from build123d import *

# Parameters (mm, degrees)
SKETCH1_W               = 63.5
SKETCH1_H               = 63.5
BOSS_EXTRUDE1_DEPTH     = 5
SKETCH2_W               = 36.5
SKETCH2_H               = 36.5
SKETCH2_W_2             = 26.5
SKETCH2_H_2             = 26.5
BOSS_EXTRUDE2_DEPTH     = 60
SKETCH13_W              = 13.5
SKETCH13_H              = 4
BOSS_EXTRUDE3_DEPTH     = 60
CUT_EXTRUDE1_DEPTH      = 81.059680864
CUT_EXTRUDE1_DEPTH_BACK = 81.059680864
SKETCH15_W              = 13.5
SKETCH15_H              = 4
BOSS_EXTRUDE4_DEPTH     = 60
CUT_EXTRUDE3_DEPTH      = 81.059680864
CUT_EXTRUDE3_DEPTH_BACK = 81.059680864
SKETCH17_W              = 4
SKETCH17_H              = 13.5
BOSS_EXTRUDE5_DEPTH     = 60
CUT_EXTRUDE4_DEPTH      = 81.188668152
CUT_EXTRUDE4_DEPTH_BACK = 81.188668152
SKETCH21_R              = 3.175
CUT_EXTRUDE7_DEPTH      = 20


with BuildPart() as part:
    # Sketch1 → Boss-Extrude1 (new body)
    with BuildSketch(Plane(origin=(0, 0, 0), x_dir=(1, 0, 0), z_dir=(0, 1, 0))):
        Rectangle(SKETCH1_W, SKETCH1_H)
    extrude(amount=BOSS_EXTRUDE1_DEPTH)

    # Sketch2 → Boss-Extrude2 (add)
    with BuildSketch(Plane(origin=(0, 5, 0), x_dir=(1, 0, 0), z_dir=(0, 1, 0))):
        Rectangle(SKETCH2_W, SKETCH2_H)
        Rectangle(SKETCH2_W_2, SKETCH2_H_2, mode=Mode.SUBTRACT)
    extrude(amount=BOSS_EXTRUDE2_DEPTH)

    # Sketch13 → Boss-Extrude3 (add)
    with BuildSketch(Plane(origin=(0, 5, 0), x_dir=(1, 0, 0), z_dir=(0, 1, 0))):
        with Locations((-25, -0.55)):
            Rectangle(SKETCH13_W, SKETCH13_H)
    extrude(amount=BOSS_EXTRUDE3_DEPTH)

    # Sketch14 → Cut-Extrude1 (cut, two sides: drawn at the far end of the back side and taken through both)
    with BuildSketch(Plane.XY.offset(2.55).offset(-CUT_EXTRUDE1_DEPTH_BACK)):
        Polygon((-72.29949978, -175.219999022), (-31.75, 5), (-18.25, 65), (22.29949978, 245.219999022), (-338.140498264, 326.318998582), (-432.739497824, -94.120999462), align=None)
    extrude(amount=CUT_EXTRUDE1_DEPTH + CUT_EXTRUDE1_DEPTH_BACK, mode=Mode.SUBTRACT)

    # Sketch15 → Boss-Extrude4 (add)
    with BuildSketch(Plane(origin=(0, 5, 0), x_dir=(1, 0, 0), z_dir=(0, 1, 0))):
        with Locations((25, -0.55)):
            Rectangle(SKETCH15_W, SKETCH15_H)
    extrude(amount=BOSS_EXTRUDE4_DEPTH)

    # Sketch16 → Cut-Extrude3 (cut, two sides: drawn at the far end of the back side and taken through both)
    with BuildSketch(Plane.XY.offset(2.55).offset(-CUT_EXTRUDE3_DEPTH_BACK)):
        Polygon((72.29949978, -175.219999022), (31.75, 5), (18.25, 65), (-22.29949978, 245.219999022), (338.140498264, 326.318998582), (432.739497824, -94.120999462), align=None)
    extrude(amount=CUT_EXTRUDE3_DEPTH + CUT_EXTRUDE3_DEPTH_BACK, mode=Mode.SUBTRACT)

    # Sketch17 → Boss-Extrude5 (add)
    with BuildSketch(Plane(origin=(0, 5, 0), x_dir=(1, 0, 0), z_dir=(0, 1, 0))):
        with Locations((-0.85, -25)):
            Rectangle(SKETCH17_W, SKETCH17_H)
    extrude(amount=BOSS_EXTRUDE5_DEPTH)

    # Sketch18 → Cut-Extrude4 (cut, two sides: drawn at the far end of the back side and taken through both)
    with BuildSketch(Plane.ZY.offset(2.85).offset(-CUT_EXTRUDE4_DEPTH_BACK)):
        Polygon((72.29949978, -175.219999022), (31.75, 5), (18.25, 65), (-22.29949978, 245.219999022), (338.140498264, 326.318998582), (432.739497824, -94.120999462), align=None)
    extrude(amount=CUT_EXTRUDE4_DEPTH + CUT_EXTRUDE4_DEPTH_BACK, mode=Mode.SUBTRACT)

    # Sketch21 → Cut-Extrude7 (cut)
    with BuildSketch(Plane(origin=(0, 0, -18.25), x_dir=(-1, 0, 0), z_dir=(0, 0, -1))):
        with Locations((0, 17.739365868)):
            Circle(SKETCH21_R)
        with Locations((0, 47.466444019)):
            Circle(SKETCH21_R)
    extrude(amount=-CUT_EXTRUDE7_DEPTH, mode=Mode.SUBTRACT)


solid = part.part
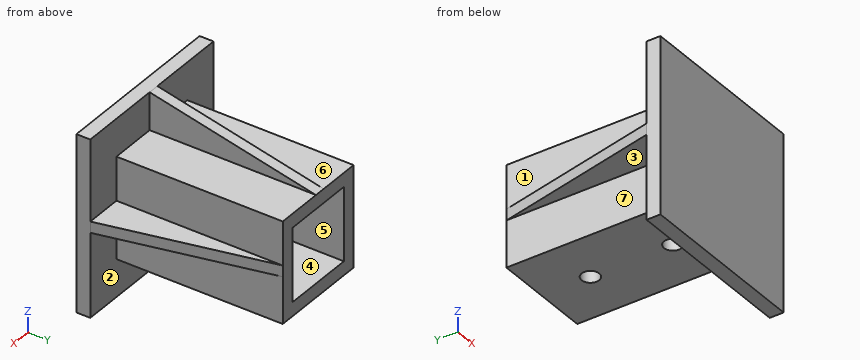
Source: CAD feature listing. Evaluate the final solid. Frame: model axes, mm. Face numbers are marked on the shaded views. A direction names the side the tool comes from. Give positions to 0.01 mm unless a question says otherwise; leave off trailing zeros. Write each loop counter-clockwise with the first axis right and the second up, starting at its lowest first coordinate (ties: lowest second). Pieces come first, ordered by that corner, then holes. Notation, with made-up numbers: M 73.25,4.25 L 120.25,4.25 A14 cw 120.25,26.25 Z; hole C 42,70 d10. An arc over 180 degrees is marked long. Answer as a JSON object with one key per item and string values.
Q1. Ray query, line 1 along Y through (x, z) = (0, -14); line 2 along X through (y, z) = (34, 12). Return the intervals inside material, ascending.
Geometry check:
{"line 1": "y = 0 to 14.56, 20.91 to 44.29, 50.64 to 65", "line 2": "x = -18.25 to -13.25, 13.25 to 18.25"}
Q2. Cut plane C-C, the plane z = -12. Return the cut outline in (x, y).
Geometry check:
{"outline": "M -31.75,0 L 31.75,0 L 31.75,5 L 18.25,5 L 18.25,65 L 13.25,65 L 13.25,5 L -13.25,5 L -13.25,65 L -18.25,65 L -18.25,5 L -31.75,5 Z"}
Q3. Access query for the marked faces 1, 2, 3 and 4. Directions: +Z, -Z, +X, -X, +Y, -Y. A direction counts if a zero-diameter tool reaches every point of the face in a straight line with its end or side. Return the directions, or none.
Geometry check:
{"face 1": "+Z, -X, +Y", "face 2": "-Z, +Y", "face 3": "-Z, -X, +Y", "face 4": "+Y"}
Q4. Cut plane B-B, the plane x = -16.5. Return the cut outline in (y, z), then the cut area to 3 significant figures.
Geometry check:
{"outline": "M 0,-31.75 L 5,-31.75 L 5,-18.25 L 65,-18.25 L 65,18.25 L 5,18.25 L 5,31.75 L 0,31.75 Z", "area": "2,510 mm^2"}
Q5. Cut plane A-A, the plane y = 41. Return the cut outline in (x, z).
Geometry check:
{"outline": "M -23.65,-1.45 L -18.25,-1.45 L -18.25,-18.25 L 18.25,-18.25 L 18.25,-1.45 L 23.65,-1.45 L 23.65,2.55 L 18.25,2.55 L 18.25,18.25 L 1.15,18.25 L 1.15,23.65 L -2.85,23.65 L -2.85,18.25 L -18.25,18.25 L -18.25,2.55 L -23.65,2.55 Z; hole M -13.25,-13.25 L 13.25,-13.25 L 13.25,13.25 L -13.25,13.25 Z"}
Q6. Cut plane D-D, the plane x = 0. Return the cut outline in (y, z).
Geometry check:
{"outline": "M 0,-31.75 L 5,-31.75 L 5,-18.25 L 14.56,-18.25 L 14.56,-13.25 L 5,-13.25 L 5,13.25 L 65,13.25 L 65,18.25 L 5,31.75 L 0,31.75 Z; M 20.91,-18.25 L 44.29,-18.25 L 44.29,-13.25 L 20.91,-13.25 Z; M 50.64,-18.25 L 65,-18.25 L 65,-13.25 L 50.64,-13.25 Z"}
Q7. Mould query, pull axis X, two halves, no side actions, for the marked faces 5, 6 and 7. Classes: +X half, -X half, draft (parallel to the pull), parting line (faces both ways), or undercut.
Geometry check:
{"face 5": "undercut", "face 6": "draft", "face 7": "-X half"}
Q8. Contact query for flat-ended pins moving along their axis: P1, Ø4.5, axis at x = -10, y = 27, coming from the +Z side; P2, Ø21, axis at y = 38.5, z = 6.5, coming from the +X side; P3, Ø4, axis at x = -21, y = 37, coming from the -Z side. Output: stop coordinate, or through.
Geometry check:
{"P1": "stops at z = 18.25", "P2": "stops at x = 26.4", "P3": "stops at z = -1.45"}
